The figure shows three views and two pictorial views of one solid part (mm, origin at its lowest corner). Answer the questions. A direction names the side the tool comes from. Round coordinates to 2 decimals unless told otherwise and drop trailing zeros. Order: outer loops, then holes, each group sorted by start corner. A loop starts at its lowest first (then second) coordinate and runs counter-clockwise, first axis right, second up. Notation, with made-up numbers: M 2.25,17 L 41.25,17 A22 ccw 41.25,33 Z; hole C 27.25,36.5 d9. An arc over 180 degrees is marked long. Return JSON: item names as keys, results as strings.
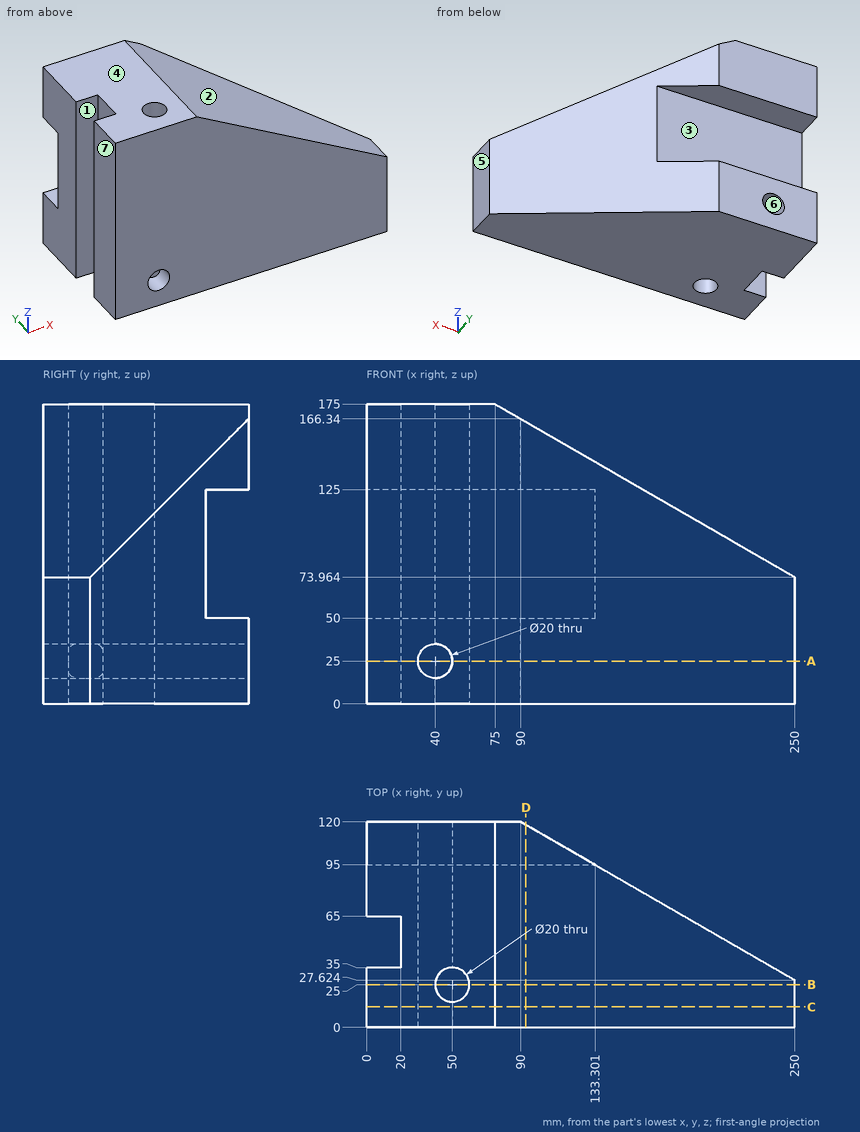
Item 1: Find section B-B (y = 25). Determine the outline of the cut face in (x, z).
Output:
{"outline": "M 0,0 L 40,0 L 40,15 A10 cw 40,35 L 40,175 L 0,175 Z; M 60,0 L 250,0 L 250,73.96 L 75,175 L 60,175 Z"}
Item 2: Consider line 1 along Y through (x, z) = (50, 137); line 2 along Y through (x, z) = (50, 74); line 3 along Z through (x, y) = (40, 90.5). Determine where each line is inside the solid, lowest interval first. Write a range as [from, to].
Output:
{"line 1": "y = [0, 15], [35, 120]", "line 2": "y = [0, 15], [35, 95]", "line 3": "z = [0, 15], [35, 175]"}
Item 3: Find section C-C (y = 12). Determine the outline of the cut face in (x, z).
Output:
{"outline": "M 0,0 L 250,0 L 250,73.96 L 75,175 L 0,175 Z; hole C 40,25 d20"}
Item 4: Each of these flat-tipped pins is pushed along its axis until it touches: pin 1 (4 mm diameter, centred on y = 59.5, z = 53, fed in from +X) (1 decimal); pin 2 (12 mm diameter, centred on x = 50, y = 25, fed in from +Z); pin 3 (7.5 mm diameter, centred on x = 96.5, y = 107, fed in from +Z); pin 4 (9 mm diameter, centred on y = 47, z = 72.5, fed in from -X). Where does it stop, or does it pass through?
Output:
{"pin 1": "stops at x = 198.3", "pin 2": "passes through", "pin 3": "stops at z = 164.75", "pin 4": "stops at x = 20"}
Item 5: The mould has two halves that part along X. Classify the marked faces 4, 5, 6 and 7: pulls with the +X half, pulls with the -X half, needs draft (parallel to the pull), parting line crosses it, or undercut.
Output:
{"face 4": "needs draft", "face 5": "pulls with the +X half", "face 6": "undercut", "face 7": "pulls with the -X half"}
Item 6: Which of the six approach directions +Z, -Z, +X, -X, +Y, -Y give full straight-line access (tool end or side, diameter ignored) to the marked faces 1, 2 and 3?
Output:
{"face 1": "+Z, -Z, -X", "face 2": "+Z, +X, +Y, -Y", "face 3": "+X, -X, +Y"}
Item 7: Find section A-A (z = 25). Determine the outline of the cut face in (x, y).
Output:
{"outline": "M 0,0 L 30,0 L 30,120 L 0,120 L 0,65 L 20,65 L 20,35 L 0,35 Z; M 50,0 L 250,0 L 250,27.62 L 90,120 L 50,120 L 50,35 A10 cw 50,15 Z"}
Item 8: Find section D-D (x = 93). Determine the outline of the cut face in (y, z).
Output:
{"outline": "M 0,0 L 118.27,0 L 118.27,50 L 95,50 L 95,125 L 118.27,125 L 118.27,164.61 L 0,164.61 Z"}
